Check sheet for the drawn part. Datum: minimum x, y, z corner. Units: mm. Give positions to 0.01 mm unless a question says otherwise; leave off trailing zeros. Order: outer loops, then holes, each group sorted by start corner. A loop starts at its lowest first (then second) coordinate and runs counter-clockwise, first axis right, second up.
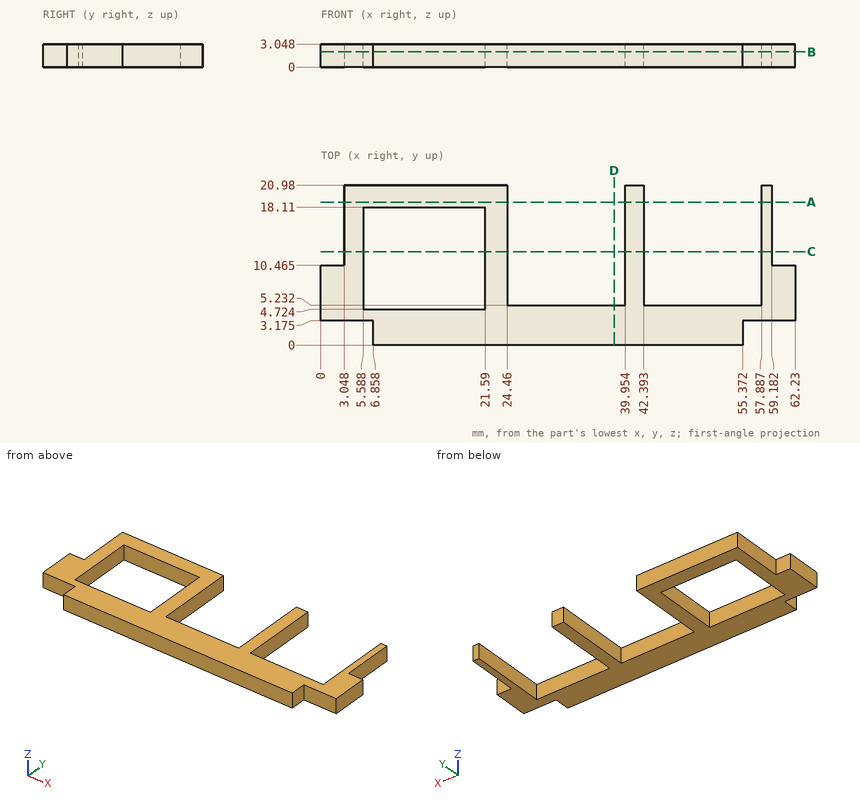
Q1. Sectioned sample at D-D, the plane x = 38.5. Record the cut outline in (y, z).
Q2. Sectioned sample at C-C, the plane y = 12.25. Record the cut outline in (x, z) (1 decimal).
Q3. Sectioned sample at B-B, the plane z = 2. Record the cut outline in (x, y) (1 decimal).
Q4. Sectioned sample at A-A, the plane y = 18.75. Record the cut outline in (x, z) (1 decimal).
Q5. Material ranges on line 1 (X direction, y = 11.25, z = 0.85) (1 decimal); line 2 (X direction, y = 8.25, z = 2.8) (1 decimal); line 3 (Y direction, x = 6.5, z = 0.3) (1 decimal), recorded low to high.
Q6. Go/stop test with flat-tipped pins: P1, Ø0.9, axis at y = 14.5, z = 2, coming from the -X side; P2, Ø0.9, axis at y = 1.5, z = 2, coming from the +X side; P3, Ø6, axis at x = 26, y = 12.5, coming from the +Z side; P4, Ø0.9, axis at x = 1.5, z = 1, coming from the +Y side (1 decimal). Record where each tip stops, or that it passes through.
Filled in:
1. outline: (0, 0) - (5.23, 0) - (5.23, 3.05) - (0, 3.05) - close
2. outline: (3, 0) - (5.6, 0) - (5.6, 3) - (3, 3) - close; (21.6, 0) - (24.5, 0) - (24.5, 3) - (21.6, 3) - close; (40, 0) - (42.4, 0) - (42.4, 3) - (40, 3) - close; (57.9, 0) - (59.2, 0) - (59.2, 3) - (57.9, 3) - close
3. outline: (0, 3.2) - (6.9, 3.2) - (6.9, 0) - (55.4, 0) - (55.4, 3.2) - (62.2, 3.2) - (62.2, 10.5) - (59.2, 10.5) - (59.2, 21) - (57.9, 21) - (57.9, 5.2) - (42.4, 5.2) - (42.4, 21) - (40, 21) - (40, 5.2) - (24.5, 5.2) - (24.5, 21) - (3, 21) - (3, 10.5) - (0, 10.5) - close; hole (5.6, 4.7) - (21.6, 4.7) - (21.6, 18.1) - (5.6, 18.1) - close
4. outline: (3, 0) - (24.5, 0) - (24.5, 3) - (3, 3) - close; (40, 0) - (42.4, 0) - (42.4, 3) - (40, 3) - close; (57.9, 0) - (59.2, 0) - (59.2, 3) - (57.9, 3) - close
5. line 1: x = 3 to 5.6, 21.6 to 24.5, 40 to 42.4, 57.9 to 59.2
5. line 2: x = 0 to 5.6, 21.6 to 24.5, 40 to 42.4, 57.9 to 62.2
5. line 3: y = 3.2 to 4.7, 18.1 to 21
6. P1: stops at x = 3.05
6. P2: stops at x = 55.37
6. P3: stops at z = 3.05
6. P4: stops at y = 10.5
